```python
from build123d import *

# Parameters (mm, degrees)
SKETCH1_W                 = 25.4
SKETCH1_H                 = 50.8
SKETCH1_W_2               = 20.32
SKETCH1_H_2               = 45.72
BOSS_EXTRUDE1_DEPTH       = 127
SKETCH2_R                 = 2.032
CUT_EXTRUDE1_DEPTH        = 138.371503595
SKETCH3_R                 = 14.3002
CUT_EXTRUDE2_DEPTH        = 132.982271537
CUT_EXTRUDE3_REACH        = 133.982
SKETCH4_W                 = 50.8
SKETCH4_H                 = 25.4
F_8_32_TAPPED_HOLE1_D     = 3.4544
F_8_32_TAPPED_HOLE1_DEPTH = 2.54


with BuildPart() as part:
    # Sketch1 → Boss-Extrude1 (new body)
    with BuildSketch(Plane.XY):
        Rectangle(SKETCH1_W, SKETCH1_H)
        Rectangle(SKETCH1_W_2, SKETCH1_H_2, mode=Mode.SUBTRACT)
    extrude(amount=BOSS_EXTRUDE1_DEPTH)

    # Sketch2 → Cut-Extrude1 (cut, through all)
    with BuildSketch(Plane(origin=(0, 25.4, 0), x_dir=(1, 0, 0), z_dir=(0, 1, 0))):
        with Locations(Location((0, -12.7, 0), (0, 0, 270))):
            Circle(SKETCH2_R)
        with Locations(Location((0, -25.4, 0), (0, 0, 270))):
            Circle(SKETCH2_R)
        with Locations(Location((0, -38.1, 0), (0, 0, 270))):
            Circle(SKETCH2_R)
        with Locations(Location((0, -50.8, 0), (0, 0, 270))):
            Circle(SKETCH2_R)
        with Locations(Location((0, -63.5, 0), (0, 0, 270))):
            Circle(SKETCH2_R)
        with Locations(Location((0, -76.2, 0), (0, 0, 270))):
            Circle(SKETCH2_R)
        with Locations(Location((0, -88.9, 0), (0, 0, 270))):
            Circle(SKETCH2_R)
        with Locations(Location((0, -101.6, 0), (0, 0, 270))):
            Circle(SKETCH2_R)
    extrude(amount=-CUT_EXTRUDE1_DEPTH, mode=Mode.SUBTRACT)

    # Sketch3 → Cut-Extrude2 (cut, through all)
    with BuildSketch(Plane(origin=(12.7, 0, 0), x_dir=(0, 0, -1), z_dir=(1, 0, 0))):
        with Locations((-88.9, 0)):
            Circle(SKETCH3_R)
    extrude(amount=-CUT_EXTRUDE2_DEPTH, mode=Mode.SUBTRACT)

    # Sketch4 → Cut-Extrude3 (cut, up to next)
    with BuildSketch(Plane.ZY.offset(12.7), mode=Mode.PRIVATE) as cut_extrude3_sk1:
        with Locations((25.4, 12.7)):
            Rectangle(SKETCH4_W, SKETCH4_H)
    cut_extrude3_tool1 = extrude(cut_extrude3_sk1.sketch, amount=-CUT_EXTRUDE3_REACH, mode=Mode.PRIVATE) & part.part
    add(cut_extrude3_tool1.solids().sort_by_distance((-12.7, 12.7, 25.4))[0], mode=Mode.SUBTRACT)

    # #8-32 Tapped Hole1
    with Locations(Plane.ZY.offset(12.7)):
        with Locations((109.522229928, 11.90625), (109.522229928, -11.90625), (68.277770072, -11.90625), (68.277770072, 11.90625)):
            Hole(F_8_32_TAPPED_HOLE1_D / 2, depth=F_8_32_TAPPED_HOLE1_DEPTH)


solid = part.part
```
The model under review builds one solid part; all positions refer to its coordinate system, in mm. A direction names the side the tool comes from. Coordinates: 2 decimals unless noted, no trailing zeros. Write each loop counter-clockwise with the first axis right and the second up, starting at its lowest first coordinate (ties: lowest second). Pieces come first, ordered by that corner, then holes.
1) We need section A-A on z = 88.9. State the section outline as (x, y) points, then the cut area to 3 significant figures.
2) To check wall thickness, follow probe 1 along Y at (x, z) = (5, 105); probe 2 along X at (y, z) = (-24, 38); probe 3 along X at (y, z) = (-1.5, 116). State the ranges of each line that lie inside material, in increasing order.
3) The part is to be moulded in two halves that separate along Y. For faces 1 (the face through (-11.41, 13.62, 68.5)), 2 (the face through (11, 0, 25)), 3 (the face through (-11.412, -12.687, 82.301)), 4 (the face through (-0.778, -24.112, 103.477)), say which applies: pulls with the +Y half, pulls with the -Y half, needs draft (parallel to the pull), parting line crosses it, or undercut.
4) Clearance check with flat-ended pins moving along their axes: pin 1 Ø6 at (x, y) = (4.5, 6) entering from +Z; pin 2 Ø0.8 at (x, z) = (11, 29) entering from +Y; pin 3 Ø1 at (x, y) = (-10, -13) entering from -Z. State where each tip first meets the part, or that it passes through.
5) We need section C-C on y = 9. State the section outline as (x, z) points, then the cut area to 3 significant figures.
6) We need section B-B on x = -3.25. State the section outline as (y, z) points.
7) We need section D-D on z = 38.1. State the section outline as (x, y) points.
8) Machinability: for faces 5 (the face through (-11.412, -10.194, 68.503)), 6 (the face through (0.09, 24.15, 86.87)), 7 (the face through (2, 22.86, 88)), which of the approach directions +Z, -Z, +X, -X, +Y, -Y give a long, thin tool a straight path to every point of the face, cutting with its end or side? Answer none if there is none.
Answer list:
1. outline: (-12.7, -25.4) - (-2.03, -25.4) - (-2.03, -22.86) - (-10.16, -22.86) - (-10.16, -14.3) - (-12.7, -14.3) - close; (-12.7, 14.3) - (-10.16, 14.3) - (-10.16, 22.86) - (-2.03, 22.86) - (-2.03, 25.4) - (-12.7, 25.4) - close; (2.03, -25.4) - (12.7, -25.4) - (12.7, -14.3) - (10.16, -14.3) - (10.16, -22.86) - (2.03, -22.86) - close; (2.03, 22.86) - (10.16, 22.86) - (10.16, 14.3) - (12.7, 14.3) - (12.7, 25.4) - (2.03, 25.4) - close
1. area: 195 mm2
2. probe 1: y = -25.4 to -22.86, 22.86 to 25.4
2. probe 2: x = -12.7 to -2.03, 2.03 to 12.7
2. probe 3: x = -12.7 to -10.16, 10.16 to 12.7
3. face 1: undercut
3. face 2: pulls with the +Y half
3. face 3: undercut
3. face 4: needs draft
4. pin 1: passes through
4. pin 2: stops at y = 0
4. pin 3: stops at z = 0
5. outline: (-12.7, 50.8) - (-10.16, 50.8) - (-10.16, 77.79) - (-12.7, 77.79) - close; (-12.7, 100.01) - (-10.16, 100.01) - (-10.16, 127) - (-12.7, 127) - close; (10.16, 50.8) - (12.7, 50.8) - (12.7, 77.79) - (10.16, 77.79) - close; (10.16, 100.01) - (12.7, 100.01) - (12.7, 127) - (10.16, 127) - close
5. area: 274 mm2
6. outline: (-25.4, 0) - (-22.86, 0) - (-22.86, 127) - (-25.4, 127) - close; (22.86, 50.8) - (25.4, 50.8) - (25.4, 127) - (22.86, 127) - close
7. outline: (-12.7, -25.4) - (-2.03, -25.4) - (-2.03, -22.86) - (-10.16, -22.86) - (-10.16, 0) - (-12.7, 0) - close; (2.03, -25.4) - (12.7, -25.4) - (12.7, 0) - (10.16, 0) - (10.16, -22.86) - (2.03, -22.86) - close
8. face 5: -X
8. face 6: +Y, -Y
8. face 7: +Z, -Z
